The drawing under review shows one solid part. Ordinate dimensions are in mm from its lowest x, y, z. A direction names the side the tool comes from. Give positions to 0.01 mm unless a question says otherwise; leave off trailing zeros. Loops run counter-clockwise (first coordinate to the right, second up) from the corner with the lowest first, then second, coordinate; pieces in that order, holes last. Notation, with made-up numbers: M -2,14.25 L 56,14.25 A26 ccw 56,52.25 Z; hole C 76,14 d3. An arc over 180 degrees is marked long. Answer as CSV lines item,"result".
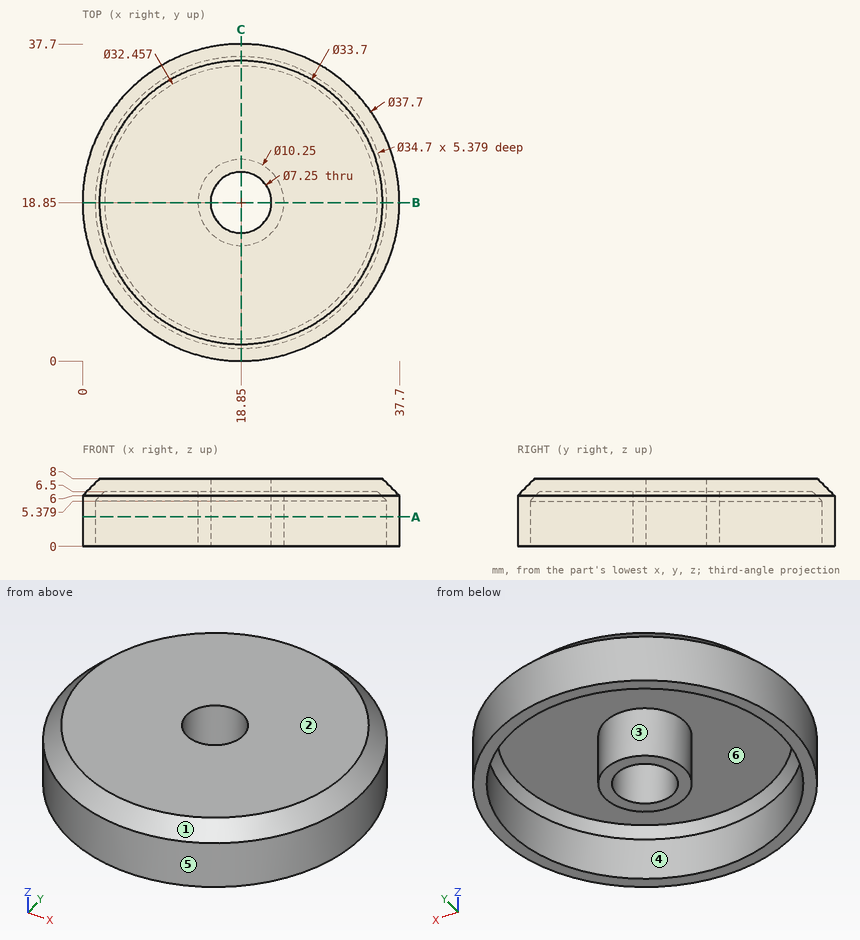
1. We need section A-A, the plane z = 3.5. Count the separate pieces of the cut face and the enclosed holes in it, plus the area to 3 significant figures.
Answer block:
separate pieces,"2"
enclosed holes,"2"
area,"212 mm²"
2. For the marked faces 5 and 6, list the 3-axis set-ups (+Z, -Z, +X, -X, +Y, -Y) from which the entire face can be reached by the end or side of a thin tool; tool diameter is ignored.
Answer block:
face 5,"+Z, -Z"
face 6,"-Z"
3. We need section B-B, the plane y = 18.85. Write out the cut boundary in (x, z) (1 decimal).
Answer block:
outline,"M 0,0 L 1.5,0 L 1.5,5.4 L 2.6,6.5 L 13.7,6.5 L 13.7,0 L 15.2,0 L 15.2,8 L 2,8 L 0,6 Z; M 22.5,0 L 24,0 L 24,6.5 L 35.1,6.5 L 36.2,5.4 L 36.2,0 L 37.7,0 L 37.7,6 L 35.7,8 L 22.5,8 Z"
4. For P1, Ø8, axis at x = 4.5, y = 5.5, coming from the +Z side; P2, Ø1, axis at x = 29, z = 1, coming from the -Y side; P3, Ø2, axis at x = 13, z = 3, coming from the -Y side (1 decimal); P4, Ø1, axis at x = 13.5, y = 25, coming from the -Z side, all flat-tipped, find the tip position at first contact; note any pin that passes through.
Answer block:
P1,"z = 8"
P2,"y = 2.66"
P3,"y = 0.6"
P4,"z = 6.5"
5. The part is to be moulded in two halves that separate along Y. For the marked faces 1, 2, 3 and 4, say which applies: pulls with the +Y half, pulls with the -Y half, needs draft (parallel to the pull), parting line crosses it, or undercut.
Answer block:
face 1,"parting line crosses it"
face 2,"needs draft"
face 3,"undercut"
face 4,"undercut"
6. To check wall thickness, follow L1, parallel to Y at x = 18.85, z = 1.6 (1 decimal); L2, parallel to X at y = 19, z = 2.75; L3, parallel to Y at x = 20, z = 3.5 (1 decimal). State the ranges of each line that lie inside material, in increasing order. Write a range as [from, to].
Answer block:
L1,"[0, 1.5], [13.7, 15.2], [22.5, 24], [36.2, 37.7]"
L2,"[0, 1.5], [13.73, 15.23], [22.47, 23.97], [36.2, 37.7]"
L3,"[0, 1.5], [13.9, 15.4], [22.3, 23.8], [36.2, 37.7]"
